Input: dimensioned drawing with shaded views. Units: mm. Origin: part minimum x, y, z. Give positions to 0.01 mm unless a question says otherwise; leave off trailing zeros. Loops run counter-clockwise (first coordinate to the right, second up) from the corner with the lowest first, then second, coordinate; pieces in that order, holes last. Notation, with made-up numbers: (75.25, -23) -> (86.25, -23) arc R18 ccw to (86.25, -17) -> close; hole circle Ø7 at (46.5, 75.5). An arc over 180 degrees is marked (long way). One line per question, with ' | ' between items. Start each with the question number.
Item 1: Material intervals for line 1 along Z through (x, y) = (70, 62); line 2 along Y through (x, z) = (81.5, 52); line 3 along Y through (x, z) = (48.5, 90.5), sorted ascending. Write a range as [from, to].
Item 2: Mould query, pull axis Y, two halves, no side actions, for the marked faces 1, 2, 3 and 4. Classes: released by +Y, released by -Y, zero draft, split by the parting line, or undercut.
Item 3: Pin query (flat end, axial travel): P1, Ø1.5, axis at y = 81.5, z = 163, coming from the -X side; P2, Ø10, axis at x = 79, z = 34, coming from the +Y side; P3, Ø3, axis at y = 57.5, z = 183, coming from the +X side. Return the tip coordinate at first contact, or that it passes through.
Item 4: Section C-C on z = 169. Return loops of the section in (x, y), then the cut area to 3 significant figures.
Item 5: Section D-D on x = 39. Return loops of the section in (y, z) (1 decimal).
Item 6: Section B-B on y = 50. Return loops of the section in (x, z).
Item 7: Section A-A on x = 51. Return loops of the section in (y, z), then the cut area to 3 significant figures.
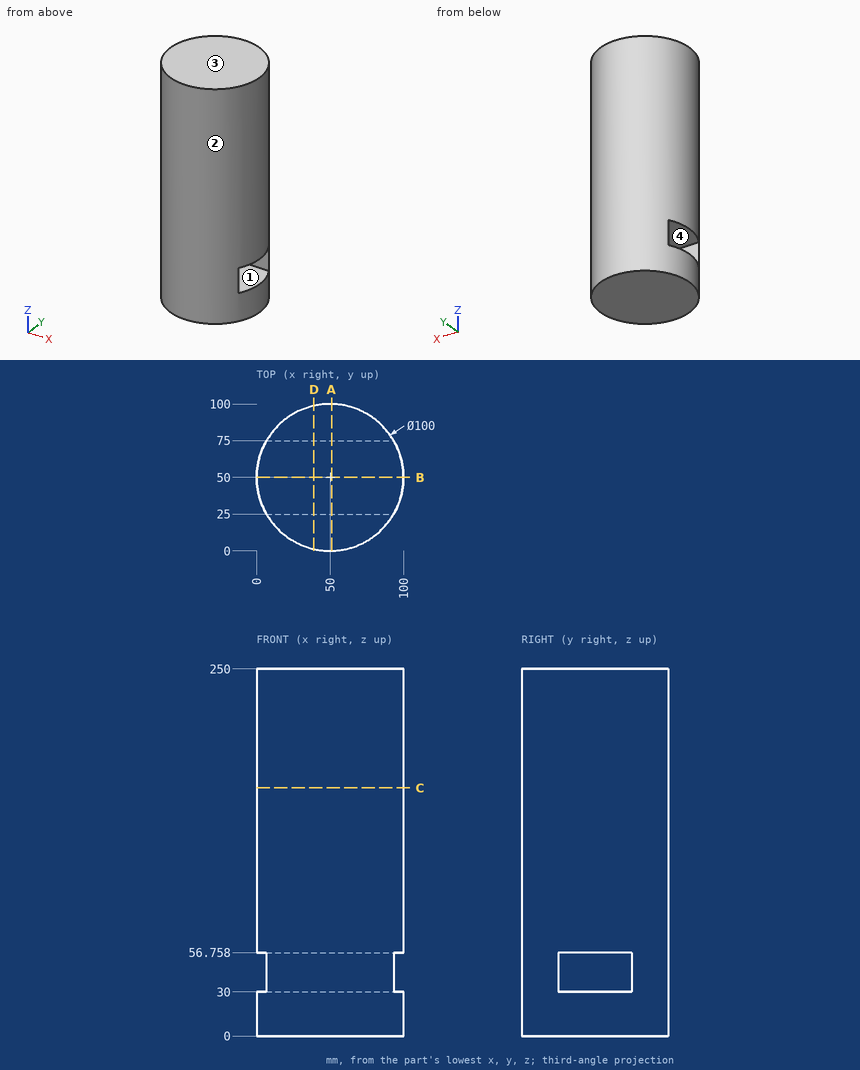
Result sheet:
1) line 1: z = [0, 30], [56.76, 250] | line 2: y = [11.17, 25], [75, 88.83] | line 3: y = [0.02, 99.98]
2) face 1: undercut | face 2: split by the parting line | face 3: zero draft | face 4: undercut
3) P1: stops at x = 10.57 | P2: stops at y = 93.86 | P3: stops at x = 99.64
4) outline: circle Ø100 at (50, 50) | area: 7,850 mm²
5) outline: (1.2, 0) -> (98.8, 0) -> (98.8, 250) -> (1.2, 250) -> close; hole (25, 30) -> (75, 30) -> (75, 56.8) -> (25, 56.8) -> close
6) outline: (0, 0) -> (100, 0) -> (100, 30) -> (0, 30) -> close; (0, 56.76) -> (100, 56.76) -> (100, 250) -> (0, 250) -> close
7) outline: (0.01, 0) -> (99.99, 0) -> (99.99, 250) -> (0.01, 250) -> close; hole (25, 30) -> (75, 30) -> (75, 56.76) -> (25, 56.76) -> close | area: 23,700 mm²
